Answer from the drawing. Dimensions are ordinates in mm from the lowest x, y and z of the part. A direction names the side the tool comes from. Coordinates: 2 decimals unless noted, no trailing zeros. Write each loop counter-clockwise with the first axis right and the second up, starting at its lowest first coordinate (ties: lowest second). Pieces come first, ordered by that corner, then holes. Notation, with made-up numbers: (3, 59.5) - (20, 59.5) arc R23 ccw to (20, 85.5) - close; hole circle Ø6 at (87.25, -20). An arc over 180 degrees is marked (long way). Use a Markdown table: item, result.
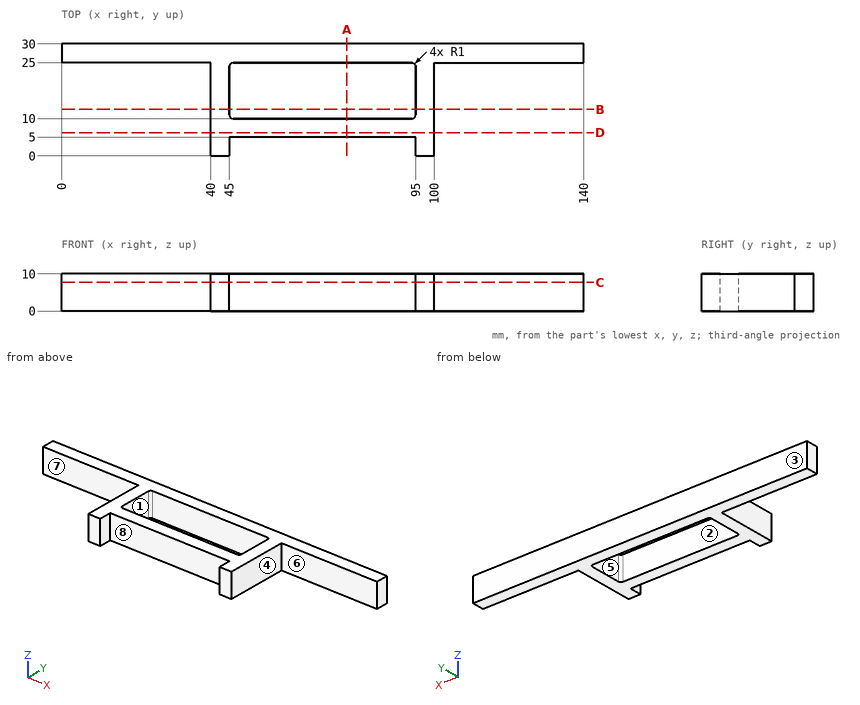
(1) A cutting plane is placed at A-A, the plane x = 76.5. Write down the section's boundary in (y, z), and give its area (3 significant figures).
Report:
| item | result |
|---|---|
| outline | (5, 0) - (10, 0) - (10, 10) - (5, 10) - close; (25, 0) - (30, 0) - (30, 10) - (25, 10) - close |
| area | 100 mm² |
(2) A cutting plane is placed at C-C, the plane z = 7.75. Write down the section's boundary in (x, y).
Report:
| item | result |
|---|---|
| outline | (0, 25) - (40, 25) - (40, 0) - (45, 0) - (45, 5) - (95, 5) - (95, 0) - (100, 0) - (100, 25) - (140, 25) - (140, 30) - (0, 30) - close; hole (45, 11) arc R1 ccw to (46, 10) - (94, 10) arc R1 ccw to (95, 11) - (95, 24) arc R1 ccw to (94, 25) - (46, 25) arc R1 ccw to (45, 24) - close |
(3) A cutting plane is placed at B-B, the plane y = 12.5. Write down the section's boundary in (x, z), and give its area (3 significant figures).
Report:
| item | result |
|---|---|
| outline | (40, 0) - (45, 0) - (45, 10) - (40, 10) - close; (95, 0) - (100, 0) - (100, 10) - (95, 10) - close |
| area | 100 mm² |
(4) Each of these flat-tipped pins is pushed along its axis until it touches: P1, Ø3, axis at y = 8, z = 5, coming from the -X side; P2, Ø3, axis at y = 15, z = 4.5, coming from the +X side; P3, Ø2, axis at x = 21, z = 4.5, coming from the -Y side. Where does it stop, or does it pass through?
Report:
| item | result |
|---|---|
| P1 | stops at x = 40 |
| P2 | stops at x = 100 |
| P3 | stops at y = 25 |
(5) Straight lines are drawn through the part: L1, parallel to Y at x = 49.5, z = 9.5; L2, parallel to X at y = 3, z = 8.5; L3, parallel to Y at x = 23.5, z = 5. For each, find the intervals that lie inside material, in ascending order.
Report:
| item | result |
|---|---|
| L1 | y = 5 to 10, 25 to 30 |
| L2 | x = 40 to 45, 95 to 100 |
| L3 | y = 25 to 30 |
(6) The mould has two halves that part along X. Classify the marked faces 1, 2, 3 and 4: pulls with the +X half, pulls with the -X half, needs draft (parallel to the pull), parting line crosses it, or undercut.
Report:
| item | result |
|---|---|
| face 1 | undercut |
| face 2 | undercut |
| face 3 | needs draft |
| face 4 | pulls with the +X half |
(7) A cutting plane is placed at D-D, the plane y = 6.25. Write down the section's boundary in (x, z), and give its area (3 significant figures).
Report:
| item | result |
|---|---|
| outline | (40, 0) - (100, 0) - (100, 10) - (40, 10) - close |
| area | 600 mm² |
(8) For the marked faces 5, 6, 7 and 8, determine the directions among +Z, -Z, +X, -X, +Y, -Y from which every point of the face is accessible in a straight line to the end or side of a thin tool.
Report:
| item | result |
|---|---|
| face 5 | +Z, -Z |
| face 6 | +Z, -Z, +X, -Y |
| face 7 | +Z, -Z, -X, -Y |
| face 8 | +Z, -Z, -Y |
